from build123d import *

# Parameters (mm, degrees)
F0_R            = 10
F1_DEPTH        = 5
F3_DEPTH        = 25
F3_COPIES_COUNT = 16
F5_R            = 5
F6_DEPTH        = 10


# Not quite as in the source:
# - a pattern or mirror of a feature is missing from the dataset's text; its kind, count and spacing are read off the source's solid


with BuildPart() as f1:
    # F0 (on Top) → F1 (new body)
    with BuildSketch(Plane.XY):
        Circle(F0_R)
    extrude(amount=F1_DEPTH)

    # F2 (on face) → F3 (cut)
    with BuildSketch(Plane.XY.offset(5)):
        with BuildLine():
            ThreePointArc((-0.9389056057, -9.9558252427), (0, -10), (0.9389056057, -9.9558252427))
            ThreePointArc((0.9389056057, -9.9558252427), (0, -9.3), (-0.9389056057, -9.9558252427))
        make_face()
    f3 = extrude(amount=-F3_DEPTH, mode=Mode.SUBTRACT)

    # F3_copies: F3 ×16 about axis
    f3_copies_axis = Axis((0, 0, 0), (0, 0, 1))
    for i in range(1, F3_COPIES_COUNT):
        add(f3.rotate(f3_copies_axis, i * 360 / F3_COPIES_COUNT), mode=Mode.SUBTRACT)

    # F5 (on face) → F6 (join)
    with BuildSketch(Plane.XY.offset(5)):
        Circle(F5_R)
        with BuildLine():
            ThreePointArc((-2.8, -1.65), (0, 3.25), (2.8, -1.65))
            Line((2.8, -1.65), (-2.8, -1.65))
        make_face(mode=Mode.SUBTRACT)
    extrude(amount=F6_DEPTH)


solid = f1.part
Could you check a few things on this model? Use its own coordinates, in mm. A direction names the side the tool comes from. Coordinates: 2 decimals unless noted, no trailing zeros. Order: outer loops, then holes, each group sorted by start corner. A loop starts at its lowest first (then second) coordinate and runs counter-clockwise, first axis right, second up.
Q1. Thinking about a two-plate mould opening in Y: for faces 1 (the cylindrical face through (-8.6, 3.54, 2.54)), 2 (the flat face through (0, -2, 15)), 3 (the cylindrical face through (8, 6, 2)), which applies, released by +Y, released by -Y, zero draft, split by the parting line, or undercut?
Q2. Suppose I cut it at D-D on z = 12. Please give me the cut outline in (x, y), and give its area (3 significant figures).
Q3. Will these pins go through, and if not, where does the flat tip stop? pin 1 (1.5 mm diameter, centred on x = 7.5, z = 4, fed in from +Y); pin 2 (3 mm diameter, centred on x = 3, z = 2.5, fed in from +Y); pin 3 (1.5 mm diameter, centred on x = -5, y = 7.5, fed in from +Z).
Q4. Which directions (+Z, -Z, +X, -X, +Y, -Y) give clear straight access to the entire face, cutting with the end or side of a thin tool? Please do faces 4 (the cylindrical face through (-6, -8, 2)), 5 (the cylindrical face through (-0.1, 3.25, 9.93)).
Q5. Please list where these lines run through material, in increasing order: L1, parallel to Y at x = 0, z = 8.25; L2, parallel to Z at x = 0.75, y = 0.75; L3, parallel to Y at x = 5.25, z = 3.25.
Q6. Suppose I cut it at B-B on y = 0. Please give me the cut outline in (x, z).
Q7. Suppose I cut it at C-C on x = 0. Please give me the cut outline in (y, z).
Answer:
1. face 1: undercut
1. face 2: zero draft
1. face 3: released by +Y
2. outline: circle Ø10 at (0, 0); hole (-2.8, -1.65) - (2.8, -1.65) arc R3.25 ccw (long way) to start
2. area: 51.7 mm2
3. pin 1: stops at y = 6.44
3. pin 2: stops at y = 9.89
3. pin 3: stops at z = 5
4. face 4: +Z, -Z, -X, -Y
4. face 5: +Z
5. L1: y = -5 to -1.65, 3.25 to 5
5. L2: z = 0 to 5
5. L3: y = -8.51 to 8.51
6. outline: (-9.3, 0) - (9.3, 0) - (9.3, 5) - (5, 5) - (5, 15) - (3.25, 15) - (3.25, 5) - (-3.25, 5) - (-3.25, 15) - (-5, 15) - (-5, 5) - (-9.3, 5) - close
7. outline: (-9.3, 0) - (9.3, 0) - (9.3, 5) - (5, 5) - (5, 15) - (3.25, 15) - (3.25, 5) - (-1.65, 5) - (-1.65, 15) - (-5, 15) - (-5, 5) - (-9.3, 5) - close
